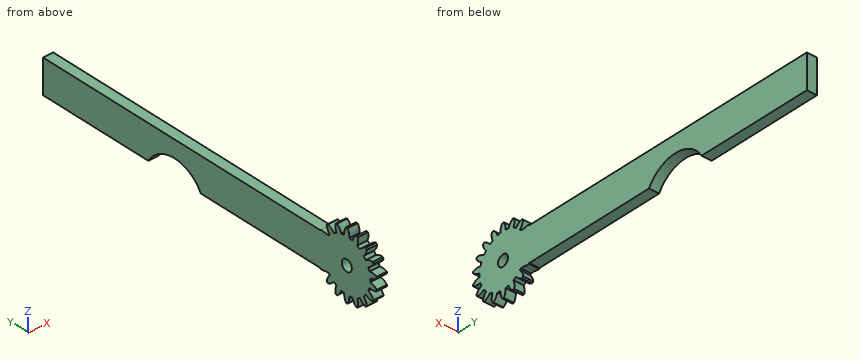
```python
from build123d import *

# Parameters (mm, degrees)
BASPROSKE_W         = 3
BASPROSKE_H         = 10
TOOTHCUT_DEPTH      = 15.456832295
TEETHCUTS_COUNT     = 18
TEETHCUTS_ANGLE     = 340
BORSKE_R            = 0.5
BORE_DEPTH          = 50.0000508
SKETCH7_W           = 10
SKETCH7_H           = 100
BOSS_EXTRUDE5_DEPTH = 3
CUT_EXTRUDE1_DEPTH  = 3
SKETCH11_R          = 1.65
CUT_EXTRUDE2_DEPTH  = 3


with BuildPart() as part:
    # BasProSke → Base-Revolve (revolve)
    with BuildSketch(Plane(origin=(0, 0, 0), x_dir=(1, 0, 0), z_dir=(0, 1, 0)), mode=Mode.PRIVATE) as base_revolve_sk:
        with Locations((1.5, 5)):
            Rectangle(BASPROSKE_W, BASPROSKE_H)
    revolve(base_revolve_sk.sketch.rotate(Axis((-10, 0, 0), (1, 0, 0)), 180), axis=Axis((-10, 0, 0), (1, 0, 0)))

    # TooCutSke → ToothCut (cut, through all)
    with BuildSketch(Plane(origin=(0, 0, 0), x_dir=(0, 0, -1), z_dir=(1, 0, 0))):
        with BuildLine():
            ThreePointArc((0.510641536, 7.732156635), (0, 7.749), (-0.510641536, 7.732156635))
            ThreePointArc((-0.510641536, 7.732156635), (-0.82619259, 8.907320741), (-1.515208602, 9.910236529))
            ThreePointArc((-1.515208602, 9.910236529), (0, 10.0254), (1.515208602, 9.910236529))
            ThreePointArc((1.515208602, 9.910236529), (0.82619259, 8.907320741), (0.510641536, 7.732156635))
        make_face()
    toothcut = extrude(amount=TOOTHCUT_DEPTH, mode=Mode.SUBTRACT)

    # TeethCuts: ToothCut ×18 about axis
    teethcuts_axis = Axis((-10, 0, 0), (1, 0, 0))
    for i in range(1, TEETHCUTS_COUNT):
        add(toothcut.rotate(teethcuts_axis, i * TEETHCUTS_ANGLE / (TEETHCUTS_COUNT - 1)), mode=Mode.SUBTRACT)

    # BorSke → Bore (cut, symmetric)
    with BuildSketch(Plane(origin=(0, 0, 0), x_dir=(0, 0, -1), z_dir=(1, 0, 0))):
        with Locations(Location((0, 0, 0), (0, 0, 180))):
            Circle(BORSKE_R)
    extrude(amount=BORE_DEPTH, both=True, mode=Mode.SUBTRACT)

    # Sketch7 → Boss-Extrude5 (add)
    with BuildSketch(Plane(origin=(3, 0, 0), x_dir=(0, 0, -1), z_dir=(1, 0, 0))):
        with Locations((0, 50)):
            Rectangle(SKETCH7_W, SKETCH7_H)
    extrude(amount=-BOSS_EXTRUDE5_DEPTH)

    # Sketch10 → Cut-Extrude1 (cut)
    with BuildSketch(Plane(origin=(3, 0, 0), x_dir=(0, 0, -1), z_dir=(1, 0, 0))):
        with BuildLine():
            Line((10, 66.692651512), (10, 46.692651512))
            ThreePointArc((10, 46.692651512), (0, 56.692651512), (10, 66.692651512))
        make_face()
    extrude(amount=-CUT_EXTRUDE1_DEPTH, mode=Mode.SUBTRACT)

    # Sketch11 → Cut-Extrude2 (cut)
    with BuildSketch(Plane.ZY):
        Circle(SKETCH11_R)
    extrude(amount=-CUT_EXTRUDE2_DEPTH, mode=Mode.SUBTRACT)


solid = part.part
```
Read the model definition and answer for the solid it produces. Units are mm, in the model's axes. Coordinates: 2 decimals unless noted, no trailing zeros. Write each loop counter-clockwise with the first axis right and the second up, starting at its lowest first coordinate (ties: lowest second). Pieces come first, ordered by that corner, then holes. Notation, with made-up numbers: (46.25, 33) -> (85.25, 33) arc R20 cw to (85.25, 42) -> close; hole circle Ø1 at (1.25, 45). An arc over 180 degrees is marked (long way). Return JSON: item names as keys, results as strings.
1. A cutting plane is placed at A-A (y = 16). Determine the outline of the cut face in (x, z), and give its area (3 significant figures).
Found:
{"outline": "(0, -5) -> (3, -5) -> (3, 5) -> (0, 5) -> close", "area": "30.0 mm2"}
2. Find the intervals of material crossed by line 1 along Y through (x, z) = (2.75, -1.25); line 2 along Y through (x, z) = (1.75, 9); line 3 along Z through (x, y) = (2.4, 9.5), in increasing order. Write a range as from..to.
Found:
{"line 1": "-9.61..-1.08, 1.08..51.85, 61.53..100", "line 2": "-3.71..-2.66, -0.71..0.71, 2.66..3.71", "line 3": "-5..5"}
3. Each of these flat-tipped pins is pushed along its axis until it touches: P1, Ø1.5, axis at x = 1.5, y = 88.5, coming from the -Z side; P2, Ø0.9, axis at x = 1, y = 6.5, coming from the +Z side. Where does it stop, or does it pass through?
Found:
{"P1": "z = -5", "P2": "z = 7.82"}
